```python
from build123d import *

# Parameters (mm, degrees)
SKIZZE1_W                                           = 35.06944
SKIZZE1_H                                           = 100
AUFSATZ_LINEAR_AUSTRAGEN1_DEPTH                     = 200
STIRNSENKUNG_F_R_M8_SENKSCHRAUBE_KOPF_B_D           = 9
STIRNSENKUNG_F_R_M8_SENKSCHRAUBE_KOPF_B_CBORE_D     = 15
STIRNSENKUNG_F_R_M8_SENKSCHRAUBE_KOPF_B_CBORE_DEPTH = 25
SPIEGELN4_COPY_1_D                                  = 9
SPIEGELN4_COPY_1_CBORE_D                            = 15
SPIEGELN4_COPY_1_CBORE_DEPTH                        = 25
KERNLOCH_F_R_M8_HELICOIL1_D                         = 8.3
KERNLOCH_F_R_M8_HELICOIL1_DEPTH                     = 20
KERNLOCH_F_R_M8_HELICOIL1_TIP                       = 2.493571569


with BuildPart() as part:
    # Skizze1 → Aufsatz-Linear austragen1 (new body)
    with BuildSketch(Plane.XY):
        Rectangle(SKIZZE1_W, SKIZZE1_H)
    extrude(amount=AUFSATZ_LINEAR_AUSTRAGEN1_DEPTH)

    # Stirnsenkung für M8 Senkschraube (Kopf Button)1 (through all)
    with Locations(Plane(origin=(17.53472, 0, 0), x_dir=(0, 0, -1), z_dir=(1, 0, 0))):
        with Locations((-165, 17.5)):
            stirnsenkung_f_r_m8_senkschraube_kopf_b = CounterBoreHole(STIRNSENKUNG_F_R_M8_SENKSCHRAUBE_KOPF_B_D / 2, STIRNSENKUNG_F_R_M8_SENKSCHRAUBE_KOPF_B_CBORE_D / 2, STIRNSENKUNG_F_R_M8_SENKSCHRAUBE_KOPF_B_CBORE_DEPTH)

    # Spiegeln3: Stirnsenkung für M8 Senkschraube (Kopf Button)1 across plane
    add(stirnsenkung_f_r_m8_senkschraube_kopf_b.mirror(Plane.XY.offset(100)), mode=Mode.SUBTRACT)

    # Spiegeln4: Stirnsenkung für M8 Senkschraube (Kopf Button)1 across plane
    add(stirnsenkung_f_r_m8_senkschraube_kopf_b.mirror(Plane.ZX), mode=Mode.SUBTRACT)

    # Spiegeln4 copy 1 (through all)
    with Locations(Plane(origin=(17.53472, 0, 200), x_dir=(0, 0, 1), z_dir=(1, 0, 0))):
        with Locations((-165, 17.5)):
            CounterBoreHole(SPIEGELN4_COPY_1_D / 2, SPIEGELN4_COPY_1_CBORE_D / 2, SPIEGELN4_COPY_1_CBORE_DEPTH)

    # Kernloch für M8 Helicoil1
    with Locations(Plane.XY.offset(200)):
        with Locations((2.53472, 0)):
            Hole(KERNLOCH_F_R_M8_HELICOIL1_D / 2, depth=KERNLOCH_F_R_M8_HELICOIL1_DEPTH)
            with Locations((0, 0, -(KERNLOCH_F_R_M8_HELICOIL1_DEPTH + KERNLOCH_F_R_M8_HELICOIL1_TIP / 2))):  # 118° drill point
                Cone(0, KERNLOCH_F_R_M8_HELICOIL1_D / 2, KERNLOCH_F_R_M8_HELICOIL1_TIP, mode=Mode.SUBTRACT)


solid = part.part
```
The listing builds one solid part. Answer for the finished solid, in the listing's coordinates (mm). A direction names the side the tool comes from. Round coordinates to 2 decimals unless told otherwise and drop trailing zeros. Loops run counter-clockwise (first coordinate to the right, second up) from the corner with the lowest first, then second, coordinate; pieces in that order, holes last. Notation, with made-up numbers: (46.25, -29) - (86.25, -29) arc R22 cw to (86.25, -1) - close; hole circle Ø9 at (58, 74). An arc over 180 degrees is marked (long way). Return JSON: item names as keys, results as strings. Group by question number.
1. The part is cut by section C-C on z = 164. Determine the outline of the cut face in (x, y).
2. Which of the six approach directions +Z, -Z, +X, -X, +Y, -Y give full straight-line access (tool end or side, diameter ignored) to faces 1 (the cylindrical face through (-1.424, 1.247, 189.86)), 2 (the flat face through (-7.465, 18, 40)), 3 (the flat face through (-4, 1, 200))?
3. Consider probe 1 along Y at (x, z) = (-11, 165); probe 2 along Z at (x, y) = (-14, -17); probe 3 along Y at (x, z) = (11.5, 35). Determine where each line is inside the solid, lowest interval first.
4. The part is cut by section B-B on y = 17.5. Determine the outline of the cut face in (x, z).
5. Each of these flat-tipped pins is pushed along its axis until it touches: P1, Ø7, axis at y = 17.5, z = 165, coming from the -X side; P2, Ø7.5, axis at y = -19, z = 167.5, coming from the +X side. Where does it stop, or does it pass through?
6. The part is cut by section A-A on x = 14.5. Determine the outline of the cut face in (y, z), then the cut area to 3 significant figures.
7. The mould has two halves that part along Y. Classify faces 4 (the cylindrical face through (-12.57, 21.294, 32.581)), 5 (the flat face through (0, 50, 99)), 6 (the conical face through (1.96, -0.44, 177.94)), 7 (the flat face through (0, 1, 0)): pulls with the +Y half, pulls with the -Y half, needs draft (parallel to the pull), parting line crosses it, or undercut.
Resolved:
{
 "1": {"outline": "(-17.53, -50) - (17.53, -50) - (17.53, -24.93) - (-7.47, -24.93) - (-7.47, -21.89) - (-17.53, -21.89) - close; (-17.53, -13.11) - (-7.47, -13.11) - (-7.47, -10.07) - (17.53, -10.07) - (17.53, 10.07) - (-7.47, 10.07) - (-7.47, 13.11) - (-17.53, 13.11) - close; (-17.53, 21.89) - (-7.47, 21.89) - (-7.47, 24.93) - (17.53, 24.93) - (17.53, 50) - (-17.53, 50) - close"},
 "2": {"face 1": "+Z", "face 2": "+X", "face 3": "+Z, +X, -X, +Y, -Y"},
 "3": {"probe 1": "y = -50 to -22, -13 to 13, 22 to 50", "probe 2": "z = 0 to 30.53, 39.47 to 160.53, 169.47 to 200", "probe 3": "y = -50 to -25, -10 to 10, 25 to 50"},
 "4": {"outline": "(-17.53, 0) - (17.53, 0) - (17.53, 27.5) - (-7.47, 27.5) - (-7.47, 30.5) - (-17.53, 30.5) - close; (-17.53, 39.5) - (-7.47, 39.5) - (-7.47, 42.5) - (17.53, 42.5) - (17.53, 157.5) - (-7.47, 157.5) - (-7.47, 160.5) - (-17.53, 160.5) - close; (-17.53, 169.5) - (-7.47, 169.5) - (-7.47, 172.5) - (17.53, 172.5) - (17.53, 200) - (-17.53, 200) - close"},
 "5": {"P1": "passes through", "P2": "stops at x = -7.47"},
 "6": {"outline": "(-50, 0) - (50, 0) - (50, 200) - (-50, 200) - close; hole circle Ø15 at (-17.5, 35); hole circle Ø15 at (-17.5, 165); hole circle Ø15 at (17.5, 35); hole circle Ø15 at (17.5, 165)", "area": "19,300 mm²"},
 "7": {"face 4": "undercut", "face 5": "pulls with the +Y half", "face 6": "undercut", "face 7": "needs draft"}
}
